Part model, mm, in its own coordinate system. A direction names the side the tool comes from. Give positions to 0.01 mm unless a question says otherwise; leave off trailing zeros. Write each loop counter-clockwise with the first axis right and the second up, starting at its lowest first coordinate (ties: lowest second). Pieces come first, ordered by that corner, then holes.
from build123d import *

# Parameters (mm, degrees)
F1_DEPTH = 6
F0_W     = 10
F0_H     = 6.1438416846
F2_DEPTH = 25
F3_DEPTH = 6
F0_R     = 2.55
F4_DEPTH = 4.4
F5_R     = 5
F7_DEPTH = 10


with BuildPart() as f1:
    # F0 (on Top) → F1 (new body)
    with BuildSketch(Plane.XY):
        with BuildLine():
            ThreePointArc((8.4852813742, -3), (0, -9), (-8.4852813742, -3))
            Line((-8.4852813742, -3), (-22.55, -3))
            Line((-22.55, -3), (-22.55, -9.1438416846))
            Line((-22.55, -9.1438416846), (22.55, -9.1438416846))
            Line((22.55, -9.1438416846), (22.55, -3))
            Line((22.55, -3), (8.4852813742, -3))
        make_face()
    extrude(amount=F1_DEPTH)

    # F0 (on Top) → F2 (join)
    with BuildSketch(Plane.XY):
        with Locations((-27.55, -6.0719208423)):
            Rectangle(F0_W, F0_H)
        with Locations((27.55, -6.0719208423)):
            Rectangle(F0_W, F0_H)
    extrude(amount=F2_DEPTH)

    # F0 (on Top) → F3 (join)
    with BuildSketch(Plane.XY):
        with BuildLine():
            ThreePointArc((-4.1243181255, -3), (-1.5773359756, 4.84994961), (5.1, 0))
            ThreePointArc((5.1, 0), (4.84994961, -1.5773359756), (4.1243181255, -3))
            Line((4.1243181255, -3), (8.4852813742, -3))
            ThreePointArc((8.4852813742, -3), (8.8703870369, -1.5219178085), (9, 0))
            ThreePointArc((9, 0), (-1.5219178085, 8.8703870369), (-8.4852813742, -3))
            Line((-8.4852813742, -3), (-4.1243181255, -3))
        make_face()
        with BuildLine():
            ThreePointArc((4.1243181255, -3), (0, -5.1), (-4.1243181255, -3))
            Line((-4.1243181255, -3), (-8.4852813742, -3))
            ThreePointArc((-8.4852813742, -3), (0, -9), (8.4852813742, -3))
            Line((8.4852813742, -3), (4.1243181255, -3))
        make_face()
    extrude(amount=F3_DEPTH)

    # F0 (on Top) → F4 (join)
    with BuildSketch(Plane.XY):
        with BuildLine():
            ThreePointArc((4.1243181255, -3), (4.84994961, -1.5773359756), (5.1, 0))
            ThreePointArc((5.1, 0), (-1.5773359756, 4.84994961), (-4.1243181255, -3))
            Line((-4.1243181255, -3), (4.1243181255, -3))
        make_face()
        Circle(F0_R, mode=Mode.SUBTRACT)
        with BuildLine():
            Line((4.1243181255, -3), (-4.1243181255, -3))
            ThreePointArc((-4.1243181255, -3), (0, -5.1), (4.1243181255, -3))
        make_face()
    extrude(amount=F4_DEPTH)

    # F5
    f5_edges = [f1.edges().sort_by_distance(p)[0] for p in [
        (-8.485281, -3, 3),
        (8.485281, -3, 3),
        (22.55, -6.071921, 6),
        (-22.55, -6.071921, 6),
        (-32.55, -6.071921, 0),
        (32.55, -6.071921, 0),
        (32.55, -6.071921, 25),
        (-32.55, -6.071921, 25),
    ]]
    fillet(f5_edges, radius=F5_R)

    # F6 (on face) → F7 (cut)
    with BuildSketch(Plane.XZ.offset(9.1438416846)):
        Polygon((17.55, 19.3), (22.55, 19.3), (22.55, 21.5), (-22.55, 21.5), (-22.55, 19.3), (-17.55, 19.3), align=None)
        Polygon((-22.55, 19.3), (-22.55, 21.5), (-24, 21.5), (-27.55, 21.5), (-27.55, 19.3), align=None)
        Polygon((22.55, 19.3), (27.55, 19.3), (27.55, 21.5), (24, 21.5), (22.55, 21.5), align=None)
        Polygon((-24, 21.5), (-22.55, 21.5), (-22.55, 25), (-27, 25), align=None)
        Polygon((22.55, 25), (22.55, 21.5), (24, 21.5), (27, 25), align=None)
        with BuildLine():
            ThreePointArc((-22.55, 19.3), (-24.654400045, 10.9190225395), (-17.55, 6))
            ThreePointArc((-17.55, 6), (-21.0855339059, 7.4644660941), (-22.55, 11))
            Line((-22.55, 11), (-22.55, 19.3))
        make_face()
        with BuildLine():
            ThreePointArc((17.55, 6), (24.654400045, 10.9190225395), (22.55, 19.3))
            Line((22.55, 19.3), (22.55, 11))
            ThreePointArc((22.55, 11), (21.0855339059, 7.4644660941), (17.55, 6))
        make_face()
    extrude(amount=-F7_DEPTH, mode=Mode.SUBTRACT)


solid = f1.part
1) Saw through at D-D (z = 18). Write the cut outline in (x, y), and give its area (3 significant figures).
Check result:
outline: (-32.55, -9.14) - (-23.73, -9.14) - (-23.73, -3) - (-32.55, -3) - close; (23.73, -9.14) - (32.55, -9.14) - (32.55, -3) - (23.73, -3) - close
area: 108 mm2
2) Mould opens along Z. For faces 1 (the cylindrical face through (31.05, -6.03, 1.43)), 2 (the flat face through (-26, -6, 21.5)), 3 (the cylindrical face through (1.18, -2.26, 2.17)) say: +Z half, -Z half, draft (parallel to the pull), parting line (faces both ways), or undercut.
Check result:
face 1: -Z half
face 2: undercut
face 3: draft
3) Saw through at A-A (x = 0). Write the cut outline in (y, z).
Check result:
outline: (-9.14, 0) - (-2.55, 0) - (-2.55, 4.4) - (-5.1, 4.4) - (-5.1, 6) - (-9.14, 6) - close; (2.55, 0) - (9, 0) - (9, 6) - (5.1, 6) - (5.1, 4.4) - (2.55, 4.4) - close
4) Flat gauge pins, fed straight in: P1, Ø15, axis at x = -24.5, z = 18, coming from the +Y side; P2, Ø6, axis at x = 14, y = 0.5, coming from the -Z side; P3, Ø6, axis at x = 0.5, y = 5, coming from the +Z side; P4, Ø4, axis at x = -24, y = -6, coming from the +Z side. Where does each tip first touch, or does it go through?
Check result:
P1: stops at y = -3
P2: passes through
P3: stops at z = 6
P4: stops at z = 23.83
5) 3-axis set-ups, long thin cutter, end or side, ignore diameter. For faces 4 (the flat face through (32.55, -6, 12)), 5 (the flat face through (0, -6, 6)), 6 (the flat face through (2, -2, 4.4)), 7 (the flat face through (-25, -3, 10)), 8 (the flat face through (-25, -6, 19.3)): which of +Z, -Z, +X, -X, +Y, -Y reach the whole face in a straight line?
Check result:
face 4: +Z, -Z, +X, +Y, -Y
face 5: +Z, +Y, -Y
face 6: +Z
face 7: +Z, -Z, -X, +Y
face 8: +Y, -Y
6) Saw through at C-C (y = -6.25). Write the cut outline in (x, z), and give its area (3 significant figures).
Check result:
outline: (-32.55, 5) arc R5 ccw to (-27.55, 0) - (27.55, 0) arc R5 ccw to (32.55, 5) - (32.55, 20) arc R5 ccw to (27.55, 25) - (27, 25) - (24, 21.5) - (27.55, 21.5) - (27.55, 19.3) - (22.55, 19.3) arc R7.59 cw to (17.55, 6) - (-17.55, 6) arc R7.59 cw to (-22.55, 19.3) - (-27.55, 19.3) - (-27.55, 21.5) - (-24, 21.5) - (-27, 25) - (-27.55, 25) arc R5 ccw to (-32.55, 20) - close
area: 671 mm2
7) Drill centre lines: L1, parallel to Z at x = 14, y = -6; L2, parallel to Y at x = -29, z = 5.5; L3, parallel to Z at x = 23, y = -7. Where is each one in solid material? Low to high.
Check result:
L1: z = 0 to 6
L2: y = -9.14 to -3
L3: z = 0 to 8.31, 18.87 to 19.3
8) Saw through at B-B (z = 22.5). Write the cut outline in (x, y).
Check result:
outline: (-31.88, -9.14) - (-24.86, -9.14) - (-24.86, -3) - (-31.88, -3) - close; (24.86, -9.14) - (31.88, -9.14) - (31.88, -3) - (24.86, -3) - close
